Geometry check sheet. Reference: the model listing, model coordinates, mm. A direction names the side the tool comes from. Round coordinates to 2 decimals unless told otherwise and drop trailing zeros. Order: outer loops, then holes, each group sorted by start corner. A loop starts at its lowest first (then second) coordinate and runs counter-clockwise, first axis right, second up.
(1) Go/stop test with flat-tipped pins: pin 1 (5 mm diameter, centred on x = 2, y = 3, fed in from +Z); pin 2 (1.6 mm diameter, centred on y = -5, z = 2.5, fed in from -X); pin 3 (1.5 mm diameter, centred on x = -1, y = -3, fed in from -Z); pin 4 (1.5 mm diameter, centred on x = -4, y = -2, fed in from +Z). Record where each tip stops, or that it passes through.
(2) Sectioned sample at A-A (x = -1). Record the boundary of the cut face in (y, z), plus the area to 3 significant figures.
(3) Set-up check for faces 1 (the face through (-9, 0, 3)), 2 (the face through (-9.1, 1.5, 1.6)), 3 (the face through (3, 3, 1)), 4 (the face through (-6.5, -5, 0.9)): record each of +Z, -Z, +X, -X, +Y, -Y from which the full face is reachable in a straight line by a thin tool's end or side.
(4) Sectioned sample at B-B (y = 0). Record the boundary of the cut face in (x, z).
(5) Material ranges on line 1 along Y through (x, z) = (-12, 3.25); line 2 along Y through (x, z) = (-12.5, 4.25); line 3 along Y through (x, z) = (-3.5, 2.5), recorded low to high.
(6) Release check for a two-part mould opening along Z. For faces 5 (the face through (-9.5, 0, 4.2)), 6 (the face through (-6, -0.1, 0.5)), 7 (the face through (-1.57, 4.91, 1.66)) record: +Z half, -Z half, draft (parallel to the pull), parting line (faces both ways), or undercut.
(7) Sectioned sample at D-D (x = -11.5). Record the boundary of the cut face in (y, z).
(8) Sectioned sample at C-C (x = -5). Record the boundary of the cut face in (y, z).
from build123d import *

# Parameters (mm, degrees)
SKETCH1_R             = 1.1
BOSS_EXTRUDE1_DEPTH   = 6
SKETCH2_R             = 4
CUT_EXTRUDE2_DEPTH    = 10
CUT_EXTRUDE4_START    = -6
CUT_EXTRUDE4_DEPTH    = 18.853720884
CUT_EXTRUDE6_DEPTH    = 24.853720884
CROQUIS1_W            = 1
CROQUIS1_H            = 5.5
CROQUIS1_H_2          = 10
CORTAR_EXTRUIR1_DEPTH = 18.606816862
FILLET4_R             = 3
FILLET1_SIZE          = 0.5
SKETCH5_R             = 1.75
CUT_EXTRUDE5_DEPTH    = 4
CHAFL_N1_SIZE         = 1


with BuildPart() as part:
    # Sketch1 → Boss-Extrude1 (new body)
    with BuildSketch(Plane.XY):
        with BuildLine():
            Line((-15, 7), (0, 7))
            ThreePointArc((0, 7), (7, 0), (0, -7))
            Line((0, -7), (-15, -7))
            Line((-15, -7), (-15, 7))
        make_face()
        with Locations((-12, 3.5)):
            Circle(SKETCH1_R, mode=Mode.SUBTRACT)
        with Locations(Location((-12, -3.5, 0), (0, 0, 180))):
            Circle(SKETCH1_R, mode=Mode.SUBTRACT)
    extrude(amount=BOSS_EXTRUDE1_DEPTH)

    # Sketch2 → Cut-Extrude2 (cut)
    with BuildSketch(Plane(origin=(0, 0, 0), x_dir=(-1, 0, 0), z_dir=(0, 0, -1))):
        Circle(SKETCH2_R)
    extrude(amount=-CUT_EXTRUDE2_DEPTH, mode=Mode.SUBTRACT)

    # Sketch7 → Cut-Extrude4 (cut, through all)
    with BuildSketch(Plane.ZY.offset(15).offset(CUT_EXTRUDE4_START)):
        Polygon((2.3, 5.55), (1, 4.25), (1, -4.25), (2.3, -5.55), (4.5, -5.55), (5.1, -4.95), (6, -4.95), (6, 4.95), (5.1, 4.95), (4.5, 5.55), align=None)
    extrude(amount=-CUT_EXTRUDE4_DEPTH, mode=Mode.SUBTRACT)

    # Sketch8 → Cut-Extrude6 (cut, through all)
    with BuildSketch(Plane.ZY.offset(15)):
        with BuildLine():
            Line((4.7, 1.363340016), (4.7, -1.363340016))
            ThreePointArc((4.7, -1.363340016), (4.904046985, -1.855953015), (5.396659984, -2.06))
            Line((5.396659984, -2.06), (6, -2.06))
            Line((6, -2.06), (6, 2.06))
            Line((6, 2.06), (5.396659984, 2.06))
            ThreePointArc((5.396659984, 2.06), (4.904046985, 1.855953015), (4.7, 1.363340016))
        make_face()
    extrude(amount=-CUT_EXTRUDE6_DEPTH, mode=Mode.SUBTRACT)

    # Croquis1 → Cortar-Extruir1 (cut, through all)
    with BuildSketch(Plane(origin=(0, 0, 0), x_dir=(-1, 0, 0), z_dir=(0, 0, -1))):
        with Locations((9, 4.25)):
            Rectangle(CROQUIS1_W, CROQUIS1_H)
        with Locations((6.5, 0)):
            Rectangle(CROQUIS1_W, CROQUIS1_H_2)
        with Locations((9, -4.25)):
            Rectangle(CROQUIS1_W, CROQUIS1_H)
    extrude(amount=-CORTAR_EXTRUIR1_DEPTH, mode=Mode.SUBTRACT)

    # Fillet4
    fillet4_edges = [part.edges().sort_by_distance(p)[0] for p in [
        (-15, -7, 3),
        (-15, 7, 3),
    ]]
    fillet(fillet4_edges, radius=FILLET4_R)

    # Fillet1
    fillet1_edges = [part.edges().sort_by_distance(p)[0] for p in [
        (-4.25, -7, 0),
        (-10.75, 7, 0),
        (-15, 0, 0),
        (-10.75, -7, 0),
        (-14.121320344, -6.121320344, 0),
        (-14.121320344, 6.121320344, 0),
        (-4.25, 7, 0),
        (7, 0, 0),
    ]]
    chamfer(fillet1_edges, length=FILLET1_SIZE)

    # Sketch5 → Cut-Extrude5 (cut)
    with BuildSketch(Plane.XY):
        with Locations((-12, 3.5)):
            Circle(SKETCH5_R)
        with Locations((-12, -3.5)):
            Circle(SKETCH5_R)
    extrude(amount=CUT_EXTRUDE5_DEPTH, mode=Mode.SUBTRACT)

    # Chaflán1
    chafl_n1_edges = [part.edges().sort_by_distance(p)[0] for p in [
        (-9, 0, 1),
    ]]
    chamfer(chafl_n1_edges, length=CHAFL_N1_SIZE)
    # the kernel refuses this chamfer: 1 mm, written as the material it takes off along each edge
    with BuildSketch(Plane(origin=(-9, 1.363340016, 4.7), x_dir=(0, 0, -1), z_dir=(0, -1, 0))) as chafl_n1_2_piece_1:
        with BuildLine():
            Line((1.028284271, 0.028284271), (-0.028284271, -1.028284271))
            Line((-0.028284271, -1.028284271), (-0.048284271, -1.028284271))
            ThreePointArc((-0.048284271, -1.028284271), (-0.02, -0.514142136), (-0.02, 0))
            Line((-0.02, 0), (0, 0.02))
            ThreePointArc((0, 0.02), (0.514142136, 0.02), (1.028284271, 0.048284271))
            Line((1.028284271, 0.048284271), (1.028284271, 0.028284271))
        make_face()
    extrude(amount=2.726680031, mode=Mode.SUBTRACT)
    with BuildSketch(Plane(origin=(-9, 1.363340016, 5.396659984), x_dir=(0, -0.6796769184207155, 0.7335116131092404), z_dir=(0, -0.7335116131092404, -0.6796769184207155))) as chafl_n1_2_piece_2:
        with BuildLine():
            Line((1.724944256, -0.028284271), (0.668375713, 1.028284271))
            Line((0.668375713, 1.028284271), (0.648375713, 1.028284271))
            ThreePointArc((0.648375713, 1.028284271), (0.676659984, 0.514142136), (0.676659984, 0))
            Line((0.676659984, 0), (0.696659984, -0.02))
            ThreePointArc((0.696659984, -0.02), (1.21080212, -0.02), (1.724944256, -0.048284271))
            Line((1.724944256, -0.048284271), (1.724944256, -0.028284271))
        make_face()
    revolve(axis=Axis((-9, 1.363340016, 5.396659984), (-1, 0, 0)), revolution_arc=222.818401466, mode=Mode.SUBTRACT)
    with BuildSketch(Plane(origin=(-9, -1.363340016, 5.396659984), x_dir=(0, 0, -1), z_dir=(0, 1, 0))) as chafl_n1_2_piece_3:
        with BuildLine():
            Line((1.724944256, -0.028284271), (0.668375713, 1.028284271))
            Line((0.668375713, 1.028284271), (0.648375713, 1.028284271))
            ThreePointArc((0.648375713, 1.028284271), (0.676659984, 0.514142136), (0.676659984, 0))
            Line((0.676659984, 0), (0.696659984, -0.02))
            ThreePointArc((0.696659984, -0.02), (1.21080212, -0.02), (1.724944256, -0.048284271))
            Line((1.724944256, -0.048284271), (1.724944256, -0.028284271))
        make_face()
    revolve(axis=Axis((-9, -1.363340016, 5.396659984), (-1, 0, 0)), revolution_arc=222.818401466, mode=Mode.SUBTRACT)


solid = part.part
Answer below:
1. pin 1: stops at z = 6
1. pin 2: stops at x = -14.99
1. pin 3: passes through
1. pin 4: stops at z = 1
2. outline: (-7, 0.5) - (-6.5, 0) - (-3.87, 0) - (-3.87, 1) - (-4.25, 1) - (-5.55, 2.3) - (-5.55, 4.5) - (-4.95, 5.1) - (-4.95, 6) - (-7, 6) - close; (3.87, 0) - (6.5, 0) - (7, 0.5) - (7, 6) - (4.95, 6) - (4.95, 5.1) - (5.55, 4.5) - (5.55, 2.3) - (4.25, 1) - (3.87, 1) - close
2. area: 23.6 mm2
3. face 1: +Z, +X, +Y, -Y
3. face 2: +Z, -Z, +Y
3. face 3: +Z, +X
3. face 4: +Z, -Z
4. outline: (-15, 0.5) - (-14.5, 0) - (-7, 0) - (-7, 1) - (-8, 1) - (-9, 2) - (-9, 3.7) - (-10, 4.7) - (-15, 4.7) - close; (-6, 0) - (-4, 0) - (-4, 1) - (-6, 1) - close; (4, 0) - (6.5, 0) - (7, 0.5) - (7, 1) - (4, 1) - close
5. line 1: y = -7 to -5.25, -1.75 to 1.75, 5.25 to 7
5. line 2: y = -6.96 to -4.48, -2.52 to 2.52, 4.48 to 6.96
5. line 3: y = -7 to -5.55, 5.55 to 7
6. face 5: +Z half
6. face 6: draft
6. face 7: undercut
7. outline: (-7, 0.5) - (-6.5, 0) - (-5.18, 0) - (-5.18, 4) - (-4.48, 4) - (-4.48, 6) - (-7, 6) - close; (-2.52, 4) - (-1.82, 4) - (-1.82, 0) - (1.82, 0) - (1.82, 4) - (2.52, 4) - (2.52, 6) - (2.06, 6) - (2.06, 5.4) arc R0.7 cw to (1.36, 4.7) - (-1.36, 4.7) arc R0.7 cw to (-2.06, 5.4) - (-2.06, 6) - (-2.52, 6) - close; (4.48, 4) - (5.18, 4) - (5.18, 0) - (6.5, 0) - (7, 0.5) - (7, 6) - (4.48, 6) - close
8. outline: (-7, 0.5) - (-6.5, 0) - (6.5, 0) - (7, 0.5) - (7, 6) - (4.95, 6) - (4.95, 5.1) - (5.55, 4.5) - (5.55, 2.3) - (4.25, 1) - (-4.25, 1) - (-5.55, 2.3) - (-5.55, 4.5) - (-4.95, 5.1) - (-4.95, 6) - (-7, 6) - close
